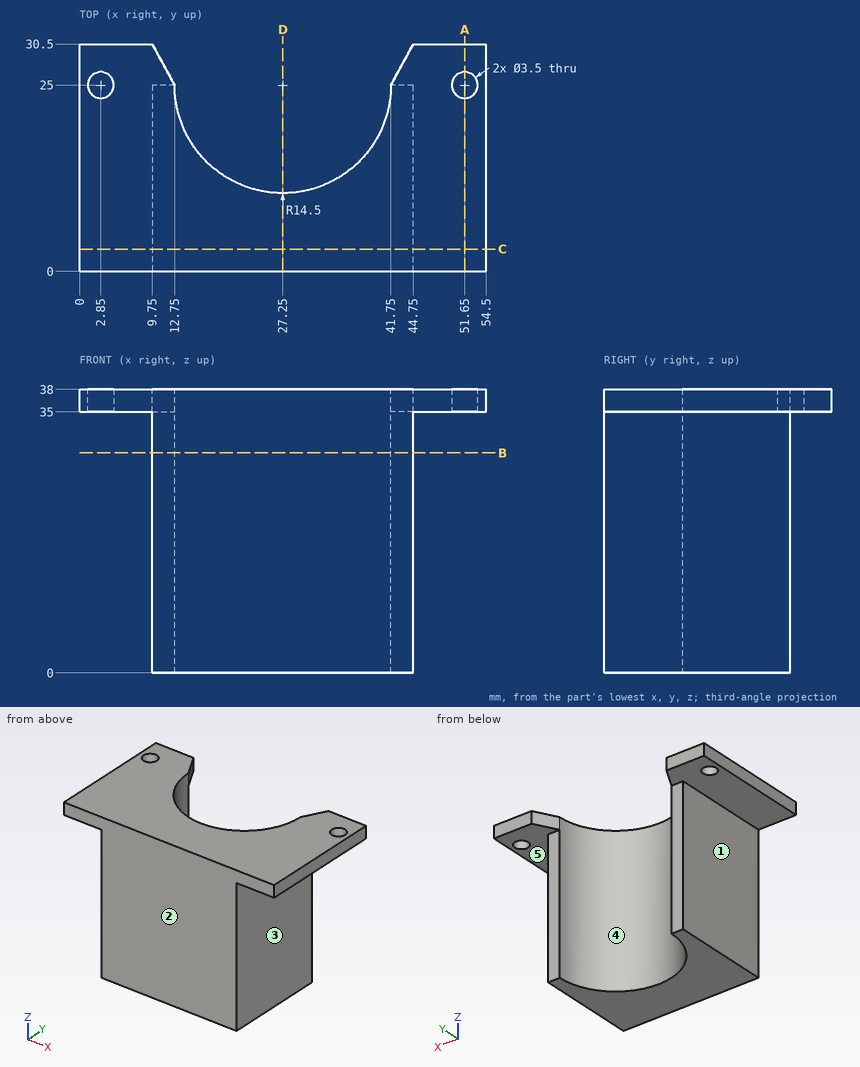
Check sheet for the drawn part. Datum: minimum x, y, z corner. Units: mm. A direction names the side the tool comes from. Round coordinates to 2 decimals unless told otherwise and drop trailing zeros. Loops run counter-clockwise (first coordinate to the right, second up) from the corner with the lowest first, then second, coordinate; pieces in that order, holes last.
Item 1: Access from +Z, -Z, +X, -X, +Y, -Y to the whole of each face (thin tool, end or side, straight path). Record for the marked faces 1 and 2.
Item 2: Gauge pin test, flat ends, axial feed: pin 1 (5 mm diameter, centred on x = 35.5, z = 21, fed in from +Y); pin 2 (7.5 mm diameter, centred on y = 15.5, z = 9.5, fed in from -X); pin 3 (4 mm diameter, centred on x = 35.5, z = 12.5, fed in from +Y). Record the tip position at first contact, or that the pin passes through.
Item 3: Cross-section at B-B on z = 29.5. Record the boundary of the cut face in (x, y).
Item 4: Mould release check, pull along X, two halves, no side actions. Record for the marked faces 3, 4 and 5: pulls with the +X half, pulls with the -X half, needs draft (parallel to the pull), parting line crosses it, or undercut.
Item 5: Cross-section at D-D on x = 27.25. Record the boundary of the cut face in (y, z), then the cut area to 3 significant figures.
Item 6: Cross-section at A-A on x = 51.65. Record the boundary of the cut face in (y, z), then the cut area to 3 significant figures.
Item 7: Cross-section at C-C on y = 3. Record the boundary of the cut face in (x, z).
Item 8: Thickness scan on line 1 (Y direction, x = 2.85, z = 35.8); line 2 (Z direction, x = 52, y = 19.5); line 3 (Y direction, x = 51, z = 36). Record the ranges inside material, lowest first.
Answer sheet:
1. face 1: -Z, -X, +Y, -Y
1. face 2: +Z, -Z, +X, -X, -Y
2. pin 1: stops at y = 15.27
2. pin 2: stops at x = 9.75
2. pin 3: stops at y = 14.74
3. outline: (9.75, 0) - (44.75, 0) - (44.75, 25) - (41.75, 25) arc R14.5 cw to (12.75, 25) - (9.75, 25) - close
4. face 3: pulls with the +X half
4. face 4: undercut
4. face 5: needs draft
5. outline: (0, 0) - (10.5, 0) - (10.5, 38) - (0, 38) - close
5. area: 399 mm2
6. outline: (0, 35) - (23.25, 35) - (23.25, 38) - (0, 38) - close; (26.75, 35) - (30.5, 35) - (30.5, 38) - (26.75, 38) - close
6. area: 81.0 mm2
7. outline: (0, 35) - (9.75, 35) - (9.75, 0) - (44.75, 0) - (44.75, 35) - (54.5, 35) - (54.5, 38) - (0, 38) - close
8. line 1: y = 0 to 23.25, 26.75 to 30.5
8. line 2: z = 35 to 38
8. line 3: y = 0 to 23.38, 26.62 to 30.5
